from build123d import *

# Parameters (mm, degrees)
SKETCH_W        = 48
SKETCH_H        = 51
PAD_DEPTH       = 8.5
POCKET_DEPTH    = 48.001
POCKET001_DEPTH = 51.001
SKETCH002_W     = 19.75
SKETCH002_H     = 40
POCKET002_DEPTH = 7
POCKET003_DEPTH = 14.5
SKETCH005_W     = 14
SKETCH005_H     = 2.5
POCKET005_DEPTH = 8.501
SKETCH007_W     = 31.75
SKETCH007_H     = 7
POCKET006_DEPTH = 1
FILLET_R        = 3
FILLET001_R     = 1
SKETCH004_R     = 1.5
SKETCH004_R_2   = 2
POCKET007_DEPTH = 5
CHAMFER_SIZE    = 0.5


with BuildPart() as part:
    # Sketch → Pad (new body)
    with BuildSketch(Plane.XY):
        Rectangle(SKETCH_W, SKETCH_H)
    extrude(amount=PAD_DEPTH)

    # Sketch006 (on Face2 of Pad) → Pocket (cut, through all)
    with BuildSketch(Plane.YZ.offset(24)):
        Polygon((25.5, 8.5), (25.5, 0), (22.75, 8.5), align=None)
    extrude(amount=-POCKET_DEPTH, mode=Mode.SUBTRACT)

    # Sketch001 (on Face3 of Pad) → Pocket001 (cut, through all)
    with BuildSketch(Plane.XZ.offset(25.5)):
        Polygon((-24, 8.5), (-24, 0), (-19, 8.5), align=None)
        Polygon((24, 8.5), (24, 0), (19, 8.5), align=None)
    extrude(amount=-POCKET001_DEPTH, mode=Mode.SUBTRACT)

    # Sketch002 → Pocket002 (cut)
    with BuildSketch(Plane(origin=(0, 0, 0), x_dir=(1, 0, 0), z_dir=(0, 0, -1))):
        with Locations((0, 5.5)):
            Rectangle(SKETCH002_W, SKETCH002_H)
    extrude(amount=-POCKET002_DEPTH, mode=Mode.SUBTRACT)

    # Sketch003 → Pocket003 (cut, symmetric)
    with BuildSketch(Plane.YZ):
        Polygon((-25.5, 3), (-25.5, 7), (14.5, 7), (14.5, 6), align=None)
    extrude(amount=POCKET003_DEPTH, both=True, mode=Mode.SUBTRACT)

    # Sketch005 → Pocket005 (cut, through all)
    with BuildSketch(Plane(origin=(0, 0, 0), x_dir=(1, 0, 0), z_dir=(0, 0, -1))):
        with Locations((0, -24.25)):
            Rectangle(SKETCH005_W, SKETCH005_H)
    extrude(amount=-POCKET005_DEPTH, mode=Mode.SUBTRACT)

    # Sketch007 (on Face2 of Pocket005) → Pocket006 (cut)
    with BuildSketch(Plane.XZ.offset(25.5)):
        with Locations((0, 3.5)):
            Rectangle(SKETCH007_W, SKETCH007_H)
    extrude(amount=-POCKET006_DEPTH, mode=Mode.SUBTRACT)

    # Fillet
    fillet_edges = [part.edges().sort_by_distance(p)[0] for p in [
        (21.5, 24.125, 4.25),
        (-21.5, 24.125, 4.25),
        (-9.875, -24.5, 1.5375),
        (9.875, -24.5, 1.5375),
    ]]
    fillet(fillet_edges, radius=FILLET_R)

    # Fillet001
    fillet001_edges = [part.edges().sort_by_distance(p)[0] for p in [
        (19, -2.705496, 8.5),
        (7, 24.25, 3.863636),
        (-7, 24.25, 3.863636),
        (-14.5, -24.5, 5.0375),
        (14.5, -24.5, 5.0375),
    ]]
    fillet(fillet001_edges, radius=FILLET001_R)

    # Sketch004 (on Face25 of Fillet001) → Pocket007 (cut)
    with BuildSketch(Plane.XY.offset(8.5)):
        with Locations((0, 6.5)):
            Circle(SKETCH004_R)
        with Locations((0, -6.5)):
            Circle(SKETCH004_R_2)
        with Locations((0, -17.5)):
            Circle(SKETCH004_R)
    extrude(amount=-POCKET007_DEPTH, mode=Mode.SUBTRACT)

    # Chamfer
    chamfer_edges = [part.edges().sort_by_distance(p)[0] for p in [
        (-2, -6.5, 8.5),
        (-1.5, -17.5, 8.5),
        (-1.5, 6.5, 8.5),
        (-1.5, -17.5, 7),
        (-2, -6.5, 7),
        (-1.5, 6.5, 7),
    ]]
    chamfer(chamfer_edges, length=CHAMFER_SIZE)


solid = part.part
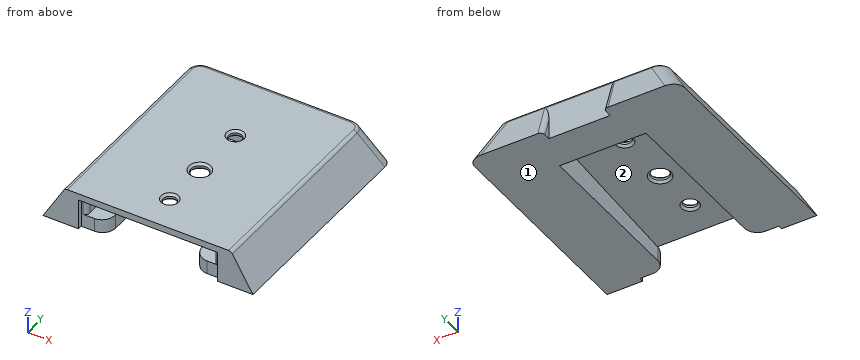
Work out the finished part from the listing and answer in its coordinate system (mm). Face numbers are marked on the shaded views. A direction names the side the tool comes from. Give positions to 0.01 mm unless a question says otherwise; leave off trailing zeros. Loops run counter-clockwise (first coordinate to the right, second up) from the corner with the lowest first, then second, coordinate; pieces in that order, holes last. Notation, with made-up numbers: (21.5, 8) - (69.5, 8) arc R14 cw to (69.5, 28) - close; hole circle Ø8 at (61.5, 8). An arc over 180 degrees is marked (long way). Answer in a Markdown table with one row per item.
(1) Section A-A (x = 0) is taken. State how many separate pieces and enclosed holes the cut face has, and give its area (3 significant figures).
Results list:
| item | result |
|---|---|
| separate pieces | 4 |
| enclosed holes | 0 |
| area | 116 mm² |
(2) Flat-ended cylindrical pins translate along their axes: pin 1 Ø1.2 at (y, z) = (24, 2.5) entering from -X; pin 2 Ø3.5 at (x, y) = (0, 6.5) entering from -Z; pin 3 Ø4 at (y, z) = (0.5, 5.5) entering from +X. Find the tip coordinate at first contact, or state that the pin passes through.
Results list:
| item | result |
|---|---|
| pin 1 | stops at x = -22.37 |
| pin 2 | stops at z = 7.25 |
| pin 3 | stops at x = 21.94 |
(3) Section C-C (x = -9) is taken. Give the vertices of the cut face in (y, z).
Results list:
| item | result |
|---|---|
| outline | (-25.5, 7) - (14.5, 7) - (14.5, 0) - (25.5, 0) - (22.97, 7.81) arc R1 ccw to (22.02, 8.5) - (-25.5, 8.5) - close |
(4) Section D-D (y = -17.5) is taken. Give the vertices of the cut face in (x, z) (3 decimals), and give its area (3 significant figures).
Results list:
| item | result |
|---|---|
| outline | (-24, 0) - (-9.875, 0) - (-9.875, 3.6) - (-14.5, 3.6) - (-14.5, 7) - (-2, 7) - (-1.5, 7.5) - (-1.5, 8) - (-2, 8.5) - (-18.428, 8.5) arc R1 ccw to (-19.29, 8.007) - close; (1.5, 7.5) - (2, 7) - (14.5, 7) - (14.5, 3.6) - (9.875, 3.6) - (9.875, 0) - (24, 0) - (19.29, 8.007) arc R1 ccw to (18.428, 8.5) - (2, 8.5) - (1.5, 8) - close |
| area | 191 mm² |
(5) A tool of negligible diameter and unlimited length cuts with its end or side. For the marked faces 1 and 2, from which of +Z, -Z, +X, -X, +Y, -Y can it reach the whole face along a straight path? Write none if from no direction.
Results list:
| item | result |
|---|---|
| face 1 | -Z, +X, -X, +Y, -Y |
| face 2 | -Y |
(6) Section B-B (y = 6.5) is taken. Give the vertices of the cut face in (x, z) (3 decimals).
Results list:
| item | result |
|---|---|
| outline | (-24, 0) - (-9.875, 0) - (-9.875, 5.4) - (-14.5, 5.4) - (-14.5, 7) - (-2, 7) - (-1.5, 7.5) - (-1.5, 8) - (-2, 8.5) - (-18.428, 8.5) arc R1 ccw to (-19.29, 8.007) - close; (1.5, 7.5) - (2, 7) - (14.5, 7) - (14.5, 5.4) - (9.875, 5.4) - (9.875, 0) - (24, 0) - (19.29, 8.007) arc R1 ccw to (18.428, 8.5) - (2, 8.5) - (1.5, 8) - close |
(7) Consider L1, parallel to Y at x = 0, z = 7.65; L2, parallel to X at y = 10, z = 3 (3 decimals); L3, parallel to Z at x = -7, y = -2. Determine where each line is inside the solid, lowest interval first. Write a range as [from, to].
Results list:
| item | result |
|---|---|
| L1 | y = [-25.5, -19], [-16, -8.5], [-4.5, 5], [8, 23] |
| L2 | x = [-22.235, -9.875], [9.875, 22.235] |
| L3 | z = [7, 8.5] |
